Autodesk Inventor part; units mm, degrees
ref_plane "YZ Plane" through (0, 0, 0) normal (1, 0, 0) x (0, 1, 0)
ref_plane "XZ Plane" through (0, 0, 0) normal (0, 1, 0) x (-1, 0, 0)
ref_plane "XY Plane" through (0, 0, 0) normal (0, 0, 1) x (1, 0, 0)
sketch "Sketch1" plane through (0, 0, 0) normal (1, 0, 0) x (0, 1, 0)
  circle A0 centre (0, 0) radius 11.684
  dimension "d0" = 23.368
extrude "Extrusion1" add sketch "Sketch1" along normal blind 33.3375
sketch "Sketch2" plane through (33.3375, 0, 0) normal (1, 0, 0) x (0, 0, -1)
  circle A0 centre (0, 0) radius 11.684
  circle A1 centre (0, 0) radius 14.2875
  dimension "d4" = 28.575
extrude "Extrusion2" add sketch "Sketch2" along normal blind 1.5875 contours A0 | A1
sketch "Sketch3" plane through (34.925, 0, 0) normal (1, 0, 0) x (0, 0, -1)
  circle A0 centre (0, 0) radius 14.2875
  line L0 (3.6662, 6.35) -> (7.3323, 0)
  line L1 (7.3323, 0) -> (3.6662, -6.35)
  line L2 (3.6662, -6.35) -> (-3.6662, -6.35)
  line L3 (-3.6662, -6.35) -> (-7.3323, 0)
  line L4 (-7.3323, 0) -> (-3.6662, 6.35)
  line L5 (-3.6662, 6.35) -> (3.6662, 6.35)
  dimension "d11" = 12.7
extrude "Extrusion3" cut sketch "Sketch3" against normal blind 50.8 contours L0 L1 L2 L3 L4 L5
chamfer "Chamfer1" distance 0.7937 angle 45 1 edges at (34.925, 0, 14.2875)
chamfer "Chamfer2" distance 1.5875 angle 45 1 edges at (0, -11.684, 0)
properties part number "colson hub" material "Aluminum 6061"
Geometry check sheet. Reference: the model listing, model coordinates, mm. A direction names the side the tool comes from. Round coordinates to 2 decimals unless told otherwise and drop trailing zeros. Write each loop counter-clockwise with the first axis right and the second up, starting at its lowest first coordinate (ties: lowest second). Pieces come first, ordered by that corner, then holes. Notation, with made-up numbers: (70, 15.25) -> (105, 15.25) arc R32 cw to (105, 43.25) -> close; hole circle Ø9 at (43, 10.25). An arc over 180 degrees is marked (long way). One line per item, written item: value. Start each with the question number.
(1) Scan lines: line 1 (Y direction, x = 33, z = 7) (3 decimals); line 2 (X direction, y = 6, z = 10.5) (1 decimal); line 3 (Z direction, x = 14, y = 2). Record each from-to range of solid material in increasing order. Write a range as [from, to].
(2) Access from +Z, -Z, +X, -X, +Y, -Y to the whole of each face (thin tool, end or side, straight path). Record for faces 1 (the flat face through (17.707, -3.131, -5.525)), 2 (the flat face through (0, 7, 0)).
(3) Cross-section at B-B, the plane x = 6. Record the cut outline in (y, z), and give its area (3 significant figures).
(4) Draft check along Z on faces 3 (the flat face through (33.338, 0, 12)), 4 (the cylindrical face through (17.24, -2.533, 11.406)), 5 (the flat face through (17.707, 3.219, -5.474)). Enter one of: +Z half, -Z half, draft (parallel to the pull), parting line (faces both ways), or undercut.
(5) Go/stop test with flat-tipped pins: pin 1 Ø6 at (x, z) = (11.5, 0) entering from +Y; pin 2 Ø10 at (x, y) = (7.5, -3) entering from -Z; pin 3 Ø1.5 at (x, z) = (30, 11) entering from -Y. Record where each tip stops, or that it passes through.
Answer:
1. line 1: [-9.355, -0.576], [0.576, 9.355]
1. line 2: [33.3, 34.9]
1. line 3: [-11.51, -6.18], [6.18, 11.51]
2. face 1: +X, -X
2. face 2: +Z, -Z, -X, +Y, -Y
3. outline: circle Ø23.37 at (0, 0); hole (-6.35, -3.67) -> (0, -7.33) -> (6.35, -3.67) -> (6.35, 3.67) -> (0, 7.33) -> (-6.35, 3.67) -> close
3. area: 289 mm²
4. face 3: draft
4. face 4: parting line
4. face 5: undercut
5. pin 1: y = 11.68
5. pin 2: z = -11.68
5. pin 3: y = -5.61
